Source: CAD feature listing. Evaluate the final solid. Frame: model axes, mm. A direction names the side the tool comes from. Round coordinates to 2 decimals unless told otherwise and drop trailing zeros. Order: outer loops, then holes, each group sorted by start corner. A loop starts at its lowest first (then second) coordinate and runs counter-clockwise, first axis right, second up. Notation, with made-up numbers: M -7,45.5 L 26,45.5 A28 cw 26,81.5 Z; hole C -29,-31 d11. An arc over 180 degrees is marked long. Answer as CSV lines item,"result". Start each with the question number.
Item 1: Pull-direction query (X, two-part tool) for faces 1 (the face through (56, -19, -22)), 2 (the face through (-1.08, -4.88, 27.58)), 3 (the face through (72.74, -38.87, 0.31)); classes: +X half, -X half, draft (parallel to the pull), parting line (faces both ways), or undercut.
Item 2: Set-up query: faces 4 (the face through (18.92, -30.88, -27.42)), 5 (the face through (18.92, -30.88, 27.42)), 6 (the face through (107.745, -38.957, 0.308)). Return all of +Z, -Z, +X, -X, +Y, -Y with unobstructed straight access to the full face (end or side cutting, diameter ignored); none if empty.
Item 3: Line query: line 1 (Z direction, x = 28, y = -39); line 2 (Y direction, x = 13, z = -7); line 3 (Y direction, x = 20.5, z = -24). Output: solid intervals per line, ascending. Write a range as [from, to].
Item 4: Section query D-D on x = 111. Return the cut outline in (y, z), plus the area to 3 significant figures.
Item 5: Section query B-B on z = -17.5. Return the cut outline in (x, y).
Item 6: Section query C-C on y = -33.5. Return the cut outline in (x, z), plus the area to 3 significant figures.
Item 7: First-contact query: P1, Ø10, axis at x = 107, z = -2, coming from the -Y side; P2, Ø6, axis at x = 83.5, z = -21, coming from the -Y side; P3, Ø12, axis at y = -22, z = 1, coming from the -X side. Flat tips, straight axial feed; report the tip coordinate or a pass-through.
Item 8: Section query A-A on z = -25. Return the cut outline in (x, y).
from build123d import *

# Parameters (mm, degrees)
ESQUISSE1_R          = 5
BASE_EXTRUSION_DEPTH = 22
ESQUISSE2_R          = 5
AXES_DEPTH           = 34
CHANFREIN1_SIZE      = 1


with BuildPart() as part:
    # Esquisse1 → Base-Extrusion (new, symmetric)
    with BuildSketch(Plane.XY):
        Polygon((0, 16.287511178), (35, 16.287511178), (160, -27), (160, -42), (125, -42), (90, -35.828555675), (55, -42), (20, -42), (-12.668949544, 0), align=None)
        Circle(ESQUISSE1_R, mode=Mode.SUBTRACT)
        with Locations((20, -26)):
            Circle(ESQUISSE1_R, mode=Mode.SUBTRACT)
    extrude(amount=BASE_EXTRUSION_DEPTH, both=True)

    # Esquisse2 → Axes (add, symmetric)
    with BuildSketch(Plane.XY):
        with Locations((20, -26)):
            Circle(ESQUISSE2_R)
        Circle(ESQUISSE2_R)
    extrude(amount=AXES_DEPTH, both=True)

    # Chanfrein1
    chanfrein1_edges = [part.edges().sort_by_distance(p)[0] for p in [
        (15, -26, -34),
        (-5, 0, -34),
        (-5, 0, 34),
        (15, -26, 34),
    ]]
    chamfer(chanfrein1_edges, length=CHANFREIN1_SIZE)


solid = part.part
Results:
1,face 1,"draft"
1,face 2,"parting line"
1,face 3,"undercut"
2,face 4,"-Z"
2,face 5,"+Z"
2,face 6,"+Z, -Z, -Y"
3,line 1,"[-22, 22]"
3,line 2,"[-33, 16.29]"
3,line 3,"[-30.97, -21.03]"
4,outline,"M -39.53,-22 L -10.03,-22 L -10.03,22 L -39.53,22 Z"
4,area,"1,300 mm^2"
5,outline,"M -12.67,0 L 20,-42 L 55,-42 L 90,-35.83 L 125,-42 L 160,-42 L 160,-27 L 35,16.29 L 0,16.29 Z"
6,outline,"M 13.39,-22 L 160,-22 L 160,22 L 13.39,22 Z"
6,area,"6,450 mm^2"
7,P1,"y = -39.71"
7,P2,"y = -37.5"
7,P3,"x = -0.22"
8,outline,"C 0,0 d10; C 20,-26 d10"
